Build history of the part. All positions in model axes, mm. A direction names the side the tool comes from. Round coordinates to 2 decimals unless told otherwise and drop trailing zeros. Loops run counter-clockwise (first coordinate to the right, second up) from the corner with the lowest first, then second, coordinate; pieces in that order, holes last.
from build123d import *

# Parameters (mm, degrees)
F1_DEPTH = 63.5
F2_DEPTH = 25.4
F3_DEPTH = 9.525
F0_W     = 12.7
F0_H     = 19.05
F0_H_2   = 15.0751015409
F0_H_3   = 16.6748984591
F5_R     = 6.35
F6_SIZE  = 5.08


with BuildPart() as f1:
    # F0 (on Front) → F1 (new body, symmetric)
    with BuildSketch(Plane.XZ):
        Polygon((-41.275, -9.525), (41.275, -9.525), (41.275, 9.525), (22.225, 9.525), (-41.275, 9.525), align=None)
    extrude(amount=F1_DEPTH, both=True)

    # F0 (on Front) → F2 (join, symmetric)
    with BuildSketch(Plane.XZ):
        with BuildLine():
            Line((22.225, 9.525), (41.275, 9.525))
            Line((41.275, 9.525), (41.275, 38.5433479412))
            ThreePointArc((41.275, 38.5433479412), (43.2187539116, 43.2359849966), (47.911390967, 45.1797389083))
            Line((47.911390967, 45.1797389083), (58.6059387632, 45.1797389083))
            Line((58.6059387632, 45.1797389083), (58.6059387632, 64.2297389083))
            Line((58.6059387632, 64.2297389083), (47.911390967, 64.2297389083))
            add(Edge.make_bspline(
                [(47.1281210154, 64.2177937793), (47.3889968052, 64.2221283934), (47.6500885902, 64.2261091673), (47.911390967, 64.2297389083)],
                knots=[104.0564336435, 104.0564336435, 104.0564336435, 104.0564336435, 104.6270557397, 104.6270557397, 104.6270557397, 104.6270557397], degree=3))
            ThreePointArc((47.1281210154, 64.2177937793), (29.473521525, 56.4272974868), (22.225, 38.5433479412))
            Line((22.225, 38.5433479412), (22.225, 9.525))
        make_face()
    extrude(amount=F2_DEPTH, both=True)

    # F0 (on Front) → F3 (join, symmetric)
    with BuildSketch(Plane.XZ):
        with BuildLine():
            add(Edge.make_bspline(
                [(-41.275, 9.525), (-40.8338249741, 50.8703959556), (-0.4441768284, 63.4273503677), (47.1281210154, 64.2177937793)],
                knots=[0, 0, 0, 0, 104.0564336435, 104.0564336435, 104.0564336435, 104.0564336435], degree=3))
            Line((-41.275, 9.525), (22.225, 9.525))
            Line((22.225, 9.525), (22.225, 38.5433479412))
            ThreePointArc((22.225, 38.5433479412), (29.473521525, 56.4272974868), (47.1281210154, 64.2177937793))
        make_face()
    extrude(amount=F3_DEPTH, both=True)

    # F0 (on Front) → F4 (revolve)
    with BuildSketch(Plane.XZ):
        with Locations((64.9559387632, 54.7047389083)):
            Rectangle(F0_W, F0_H)
        with Locations((64.9559387632, 71.7672896787)):
            Rectangle(F0_W, F0_H_2)
        with Locations((64.9559387632, 36.8422896787)):
            Rectangle(F0_W, F0_H_3)
    revolve(axis=Axis((58.6059387632, 0, 53.9048404491), (0, 0, 1)))

    # F5
    f5_edges = [f1.edges().sort_by_distance(p)[0] for p in [
        (-41.275, -63.5, 0),
        (41.275, -63.5, 0),
        (-41.275, 63.5, 0),
        (41.275, 63.5, 0),
    ]]
    fillet(f5_edges, radius=F5_R)

    # F6
    f6_edges = [f1.edges().sort_by_distance(p)[0] for p in [
        (58.605939, -25.4, 54.704739),
        (58.605939, 25.4, 54.704739),
    ]]
    chamfer(f6_edges, length=F6_SIZE)


solid = f1.part
(1) Pin check, flat tips, straight feed: P1, Ø3, axis at x = 52, y = 18, coming from the +Z side; P2, Ø15.5, axis at x = 44, z = 31.5, coming from the +Y side; P3, Ø1.5, axis at x = 4.5, y = 4.5, coming from the +Z side. Stop position of each tip, or through.
Responses:
P1: stops at z = 64.23
P2: stops at y = 25.4
P3: stops at z = 59.42
(2) Probe line 1 (Y direction, x = -24, z = 19.5) (3 decimals); line 2 (Z direction, x = 59, y = -8.5); line 3 (X direction, y = -10, z = 20.5) (3 decimals). List the from-to ranges inside material, lowest first.
Responses:
line 1: y = -9.525 to 9.525
line 2: z = 28.5 to 79.3
line 3: x = 22.225 to 41.275
(3) Which spindle directions (+Z, -Z, +X, -X, +Y, -Y) get a long thin tool onto all of the face, cutting with end or side? Do faces 1 (the face through (58.606, 16, 55)), 2 (the face through (34, 25.4, 37)), 3 (the face through (34, -25.4, 37)), 4 (the face through (22.225, 17, 24)), 5 (the face through (29.67, -17.57, 56.63)). Say none if no direction does.
Responses:
face 1: +Z, -Z, +X, +Y
face 2: +Z, +X, -X, +Y
face 3: +Z, +X, -X, -Y
face 4: +Z, -X, +Y
face 5: +Z, -X, -Y
(4) Slice it at B-B on x = 61.5. List the corners of the cut face in (y, z), plus the area to 3 significant figures.
Responses:
outline: (-12.37, 28.5) - (12.37, 28.5) - (12.37, 79.3) - (-12.37, 79.3) - close
area: 1,260 mm2
(5) Pull direction X, two halves, no side cores. Call faces 6 (the face through (1, 36, 9.525)), 7 (the face through (70.72, 3.81, 54.26)), 8 (the face through (22.225, -18, 24)): +X half, -X half, draft (parallel to the pull), parting line (faces both ways), or undercut.
Responses:
face 6: draft
face 7: undercut
face 8: -X half
(6) Slice it at A-A on z = 73. List the corners of the cut face in (x, y).
Responses:
outline: circle Ø25.4 at (58.61, 0)
